Job drawing, mm, ordinate dimensions from the low corner. One solid piece. Coordinates: 2 decimals unless noted, no trailing zeros. Write each loop counter-clockwise with the first axis right and the second up, starting at its lowest first coordinate (ties: lowest second). Pieces come first, ordered by that corner, then holes. Notation, with made-up numbers: (2, 39.5) - (31, 39.5) arc R25 ccw to (31, 52.5) - close; hole circle Ø10 at (-6, 81.25). An arc over 180 degrees is marked (long way). Put each result on its own line as item: value. Start each with the question number.
1. Saw through at A-A, the plane z = 27.9. Write the cut outline in (x, y), plus the area to 3 significant figures.
2. Drill centre lines: L1, parallel to X at y = 1, z = 27.9; L2, parallel to X at y = 0.55, z = 29; L3, parallel to Z at x = 2.75, y = 1.3. Where is each one in solid material? Low to high. Write a range as from..to.
3. Saw through at C-C, the plane y = 0.35. Write the cut outline in (x, z), plus the area to 3 significant figures.
4. Saw through at B-B, the plane x = 2.75. Write the cut outline in (y, z), plus the area to 4 significant figures.
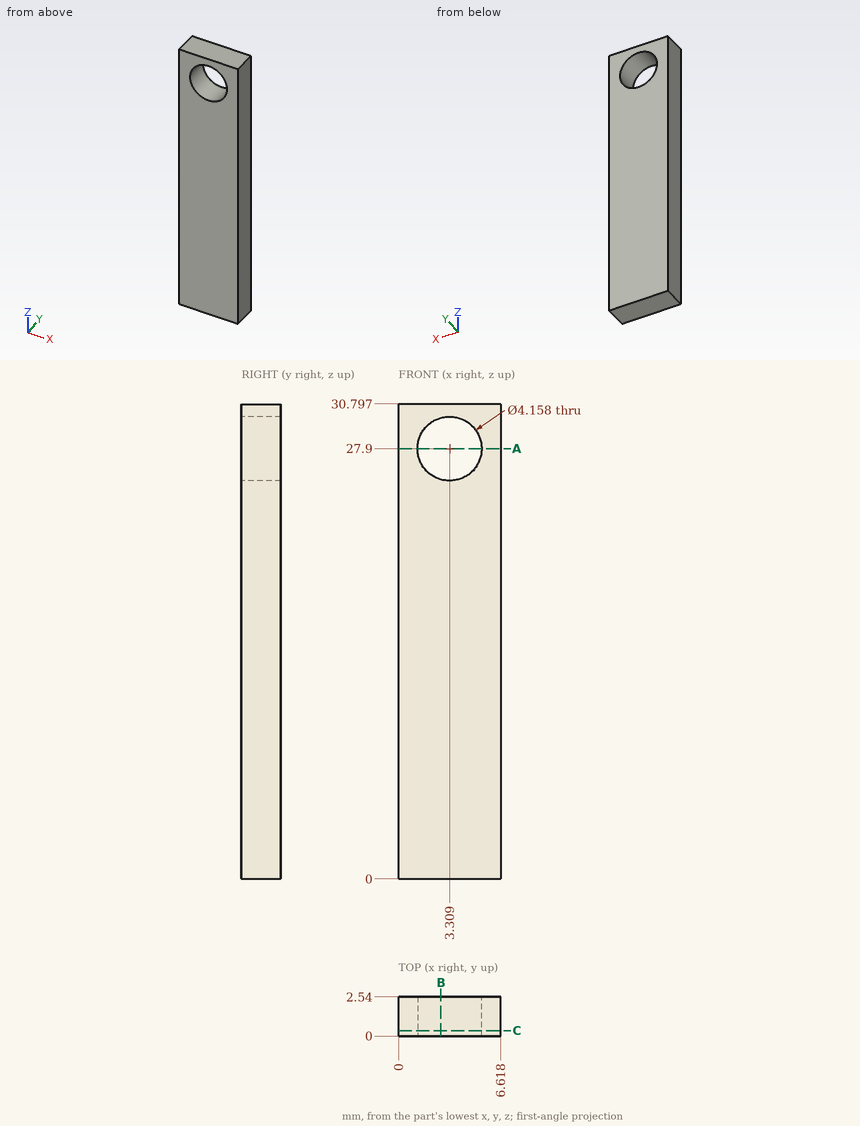
Final values:
1. outline: (0, 0) - (1.23, 0) - (1.23, 2.54) - (0, 2.54) - close; (5.39, 0) - (6.62, 0) - (6.62, 2.54) - (5.39, 2.54) - close
1. area: 6.25 mm²
2. L1: x = 0..1.23, 5.39..6.62
2. L2: x = 0..1.54, 5.07..6.62
2. L3: z = 0..25.9, 29.9..30.8
3. outline: (0, 0) - (6.62, 0) - (6.62, 30.8) - (0, 30.8) - close; hole circle Ø4.16 at (3.31, 27.9)
3. area: 190 mm²
4. outline: (0, 0) - (2.54, 0) - (2.54, 25.9) - (0, 25.9) - close; (0, 29.9) - (2.54, 29.9) - (2.54, 30.8) - (0, 30.8) - close
4. area: 68.05 mm²
